```python
from build123d import *

# Parameters (mm, degrees)
F1_DEPTH = 12.7
F2_R     = 5
F3_R     = 1.5
F4_DEPTH = 19.1


with BuildPart() as f1:
    # F0 (on Front) → F1 (new body)
    with BuildSketch(Plane.XZ):
        with BuildLine():
            Line((9.34, 0), (39.4412088344, 0))
            Line((39.4412088344, 0), (39.4394582065, 9.3399980128))
            Line((39.4394582065, 9.3399980128), (0, 9.34))
            ThreePointArc((0, 9.34), (6.6043773363, 6.6043773363), (9.34, 0))
        make_face()
        with BuildLine():
            Line((0, 9.34), (39.4394582065, 9.3399980128))
            add(Edge.make_bspline(
                [(-44.9675657917, 9.3399980128), (-29.6900332628, 9.339998688), (-0.1580063373, 15.8879383906), (26.3566872689, 9.339998672), (39.4394582065, 9.3399980128)],
                knots=[0, 0, 0, 0, 0.5162924895, 1, 1, 1, 1], degree=3))
            Line((-44.9675657917, 9.3399980128), (0, 9.34))
        make_face()
        with BuildLine():
            ThreePointArc((-9.34, 0), (-6.6043773363, 6.6043773363), (0, 9.34))
            Line((0, 9.34), (-44.9675657917, 9.3399980128))
            Line((-44.9675657917, 9.3399980128), (-44.9658151637, 0))
            Line((-44.9658151637, 0), (-9.34, 0))
        make_face()
    extrude(amount=F1_DEPTH)

    # F2
    f2_edges = [f1.edges().sort_by_distance(p)[0] for p in [
        (-44.96669, -12.7, 4.669999),
        (-44.96669, 0, 4.669999),
        (39.440334, -12.7, 4.669999),
        (39.440334, 0, 4.669999),
    ]]
    fillet(f2_edges, radius=F2_R)

    # F3 (on Top) → F4 (cut)
    with BuildSketch(Plane.XY):
        with Locations((-39.2175657917, -6.35)):
            Circle(F3_R)
        with Locations((33.6894582065, -6.35)):
            Circle(F3_R)
    extrude(amount=F4_DEPTH, mode=Mode.SUBTRACT)


solid = f1.part
```
Input: part model. Units: mm. Frame: model coordinates. Round coordinates to 2 decimals unless told otherwise and drop trailing zeros. Write each question's results on one line, items separated by ' | '.
Q1. Section query A-A (z = 1.5). State how many separate pieces and enclosed holes the cut face has, and give its area (3 significant figures).
Results:
separate pieces: 2 | enclosed holes: 2 | area: 802 mm^2
Q2. Pin query (flat end, axial travel): P1, Ø6, axis at y = -11.5, z = 6, coming from the +X side. Return the tip coordinate at first contact, or that it passes through.
Results:
P1: stops at x = 39.38
Q3. Draft query along X for faces 1 (the face through (-43.54, -11.2, 4.66)), 2 (the face through (35.12, -5.9, 4.75)), 3 (the face through (24, -6, 0)). Return one class per face: released by +X, released by -X, zero draft, split by the parting line, or undercut.
Results:
face 1: released by -X | face 2: undercut | face 3: zero draft
Q4. Line query: line 1 along Y through (x, z) = (-39, 1); line 2 along X through (y, z) = (-6.35, 5); line 3 along X through (y, z) = (-6.35, 2). Output: solid intervals per line, ascending.
Results:
line 1: y = -12.7 to -7.83, -4.87 to 0 | line 2: x = -44.97 to -40.72, -37.72 to -7.89, 7.89 to 32.19, 35.19 to 39.44 | line 3: x = -44.97 to -40.72, -37.72 to -9.12, 9.12 to 32.19, 35.19 to 39.44
